Geometry check sheet. Reference: the model listing, model coordinates, mm. A direction names the side the tool comes from. Coordinates: 2 decimals unless noted, no trailing zeros. Order: outer loops, then holes, each group sorted by start corner. A loop starts at its lowest first (then second) coordinate and runs counter-clockwise, first axis right, second up. Notation, with made-up numbers: (-27.5, -8) - (17.5, -8) arc R6 cw to (17.5, 3) - close; hole circle Ø10 at (-32.75, 9.5). An arc over 180 degrees is marked (long way). Use CSV: the item, a comma, the result in double quotes. Start each with the question number.
1) Sectioned sample at C-C, the plane y = 7.5. Record the cut outline in (x, z), and give its area (3 significant figures).
2) Sectioned sample at A-A, the plane x = -277. Record the cut outline in (y, z), and give its area (3 significant figures).
3) Tool access check on faces 1 (the cylindrical face through (-283.885, -14.79, -25.186)), 2 (the flat face through (-289, -19, 0)), 3 (the cylindrical face through (-273.983, 20.23, -23.633)), 4 (the cylindrical face through (-273.983, 4.93, -23.633)), 5 (the flat face through (-285.529, 12.613, -50.347)). Record the directions out of +Z, -Z, +X, -X, +Y, -Y that give a thin tool (end or side, any length) a straight path to the whole face; none if there is none.
4) Depth check by flat-ended pin: P1, Ø20, axis at x = -282, y = -15.5, coming from the +Z side; P2, Ø6, axis at y = 6, z = -52.5, coming from the -X side; P3, Ø6, axis at y = -19, z = -35, coming from the -X side; P4, Ø19, axis at x = -272.5, z = -29, coming from the +Y side. Enter the tip coordinate at first touch or a pass-through.
5) Sectioned sample at D-D, the plane x = -293. Record the cut outline in (y, z), and give its area (3 significant figures).
6) Draft check along Y on faces 6 (the flat face through (-284, 0, -20)), 7 (the flat face through (-278, -40, -25)), 8 (the flat face through (-287, 25.3, -27)), 9 (the cylindrical face through (-264, -35, -23)). Enter one of: released by +Y, released by -Y, zero draft, split by the parting line, or undercut.
7) Sectioned sample at B-B, the plane z = -27. Record the cut outline in (x, y), and give its area (3 significant figures).
8) Thickness scan on probe 1 along Y at (x, z) = (-276.5, -12); probe 2 along Y at (x, z) = (-296.5, -4); probe 3 along Y at (x, z) = (-298.5, 1). Record the ranges inside material, lowest first. Write a range as [from, to].
Autodesk Inventor part; units mm, degrees
ref_plane "YZ Plane" through (0, 0, 0) normal (1, 0, 0) x (0, 1, 0)
ref_plane "XZ Plane" through (0, 0, 0) normal (0, 1, 0) x (-1, 0, 0)
ref_plane "XY Plane" through (0, 0, 0) normal (0, 0, 1) x (1, 0, 0)
sketch "Sketch1" plane through (0, 0, 0) normal (0, 1, 0) x (-1, 0, 0)
  circle A0 centre (0, 0) radius 285
  circle A1 centre (0, 0) radius 295
  circle A2 centre (0, 0) radius 275
  circle A3 centre (0, 0) radius 305
  line L0 (0, 0) -> (300.3664, -52.9627)
  line L1 (0, 0) -> (305, 0)
  point P0 (275, 0)
  point P1 (270.8221, -47.7532)
  dimension "d1" = 590
  dimension "d5" = 10
  dimension "d6" = 10
  dimension "d7" = 10
  dimension "d8" = 10
extrude "Extrusion1" add sketch "Sketch1" along normal blind 10 contours L1 A1 L0 A0 | A0 L0 A2 L1 | L1 A3 L0 A1 picked at (291.5003, -5.7176) picked at (281.3509, -10.8537) picked at (297.9408, -46.5324)
sketch "Sketch2" plane through (0, 10, 0) normal (0, 1, 0) x (1, 0, 0)
  arc A0 (-270.8221, 47.7532) -> (-275, 0) centre (0, 0) ccw
  line L0 (-270.8221, 47.7532) -> (-300.3664, 52.9627)
  arc A1 (-300.3664, 52.9627) -> (-305, 0) centre (0, 0) ccw
  line L1 (-305, 0) -> (-275, 0)
  circle A2 centre (0, 0) radius 295
  circle A3 centre (0, 0) radius 285
  circle A4 centre (0, 0) radius 294.7
  circle A5 centre (0, 0) radius 285.3
  point P0 (-285, 0)
  point P1 (-280.6702, 49.4897)
  point P2 (-290.5183, 51.2262)
  point P3 (-295, 0)
  point P4 (-285.3, 0)
  point P5 (-280.9657, 49.5418)
  point P6 (-290.2228, 51.1741)
  point P7 (-294.7, 0)
  dimension "d11" = 10
  dimension "d12" = 590
  dimension "d26" = 0.3
  dimension "d27" = 0.3
extrude "Extrusion2" add sketch "Sketch2" along normal blind 5.3 contours A5 L1 A4 L0 picked at (-291.2396, 11.2413)
sketch "Sketch3" plane through (0, 15.3, 0) normal (0, 1, 0) x (1, 0, 0)
  line L0 (-290.2228, 51.1741) -> (-300.3664, 52.9627)
  arc A0 (-300.3664, 52.9627) -> (-305, 0) centre (0, 0) ccw
  line L1 (-305, 0) -> (-294.7, 0)
  line L2 (-280.9657, 49.5418) -> (-290.2228, 51.1741)
  line L3 (-294.7, 0) -> (-285.3, 0)
  line L4 (-285.3, 0) -> (-275, 0)
  arc A1 (-270.8221, 47.7532) -> (-275, 0) centre (0, 0) ccw
  line L5 (-270.8221, 47.7532) -> (-280.9657, 49.5418)
  circle A2 centre (0, 0) radius 305
  circle A3 centre (0, 0) radius 275
  line L6 (0, 0) -> (-304.7097, -13.3039)
  line L7 (0, 0) -> (-297.7703, 66.0141)
  arc A4 (-300.3664, 52.9627) -> (-305, 0) centre (0, 0) ccw
  arc A5 (-270.8221, 47.7532) -> (-275, 0) centre (0, 0) ccw
  line L8 (-290.2228, 51.1741) -> (-300.3664, 52.9627)
  line L9 (-305, 0) -> (-294.7, 0)
  line L10 (-285.3, 0) -> (-275, 0)
  line L11 (-270.8221, 47.7532) -> (-280.9657, 49.5418)
  arc A6 (-290.2228, 51.1741) -> (-294.7, 0) centre (0, 0) ccw
  arc A7 (-280.9657, 49.5418) -> (-285.3, 0) centre (0, 0) ccw
  arc A8 (-290.2228, 51.1741) -> (-294.7, 0) centre (0, 0) ccw
  arc A9 (-280.9657, 49.5418) -> (-285.3, 0) centre (0, 0) ccw
  arc A10 (-290.2228, 51.1741) -> (-294.7, 0) centre (0, 0) ccw
  arc A11 (-280.9657, 49.5418) -> (-285.3, 0) centre (0, 0) ccw
  point P0 (-270.8221, 47.7532)
  point P1 (-268.4814, 59.5209)
  point P2 (-305, 0)
  point P3 (-274.7383, -11.9953)
  point P4 (-305, 0)
  point P5 (-300.3664, 52.9627)
  point P6 (-305, 0)
  point P7 (-270.8221, 47.7532)
  dimension "d23" = 2.5
  dimension "d28" = 2.5
extrude "Extrusion3" add sketch "Sketch3" along normal blind 10 contours A6 L1 A0 L0 | L0 A2 L7 A3 L5 L2 | L2 A7 L3 A6 | L5 A1 L4 A7 | L3 L4 A3 L6 A2 L1
sketch "Sketch4" plane through (0, 0, 0) normal (0, -1, 0) x (1, 0, 0)
  arc A0 (-275, 0) -> (-270.8221, -47.7532) centre (0, 0) ccw
  line L0 (-305, 0) -> (-275, 0)
  arc A1 (-305, 0) -> (-300.3664, -52.9627) centre (0, 0) ccw
  line L1 (-270.8221, -47.7532) -> (-300.3664, -52.9627)
  circle A2 centre (0, 0) radius 285
  circle A3 centre (0, 0) radius 295
  point P0 (-295, 0)
  point P1 (-290.5183, -51.2262)
  point P2 (-280.6702, -49.4897)
  point P3 (-285, 0)
  dimension "d17" = 10
  dimension "d18" = 590
extrude "Extrusion4" add sketch "Sketch4" along normal blind 30 contours A2 L1 A3 L0 picked at (-291.3396, -11.2413)
sketch "Sketch5" plane through (0, -30, 0) normal (0, -1, 0) x (1, 0, 0)
  arc A0 (-295, 0) -> (-290.5183, -51.2262) centre (0, 0) ccw
  line L0 (-290.5183, -51.2262) -> (-280.6702, -49.4897)
  arc A1 (-285, 0) -> (-280.6702, -49.4897) centre (0, 0) ccw
  line L1 (-285, 0) -> (-295, 0)
  arc A2 (-295, 0) -> (-290.5183, -51.2262) centre (0, 0) ccw
  line L2 (-305, 0) -> (-295, 0)
  arc A3 (-305, 0) -> (-300.3664, -52.9627) centre (0, 0) ccw
  line L3 (-290.5183, -51.2262) -> (-300.3664, -52.9627)
  line L4 (-270.8221, -47.7532) -> (-280.6702, -49.4897)
  arc A4 (-275, 0) -> (-270.8221, -47.7532) centre (0, 0) ccw
  line L5 (-285, 0) -> (-275, 0)
  arc A5 (-305, 0) -> (-300.3664, -52.9627) centre (0, 0) ccw
  arc A6 (-275, 0) -> (-270.8221, -47.7532) centre (0, 0) ccw
  arc A7 (-285, 0) -> (-280.6702, -49.4897) centre (0, 0) ccw
  arc A8 (-295, 0) -> (-290.5183, -51.2262) centre (0, 0) ccw
  line L6 (-305, 0) -> (-295, 0)
  line L7 (-290.5183, -51.2262) -> (-300.3664, -52.9627)
  arc A9 (-285, 0) -> (-280.6702, -49.4897) centre (0, 0) ccw
  line L8 (-270.8221, -47.7532) -> (-280.6702, -49.4897)
  line L9 (-285, 0) -> (-275, 0)
  arc A10 (-295, 0) -> (-290.5183, -51.2262) centre (0, 0) ccw
  circle A11 centre (0, 0) radius 265
  line L10 (0, 0) -> (-305, 0)
  line L11 (0, 0) -> (-300.3664, -52.9627)
  point P0 (-290.5183, -51.2262)
  point P1 (-260.9741, -46.0168)
  point P2 (-265, 0)
  dimension "d25" = 30
extrude "Extrusion5" add sketch "Sketch5" along normal blind 10 contours L1 A1 L0 A0 | L5 A4 L4 A1 | L10 A11 L11 A4
equation "\"d27\" = d26"
equation "\"d28\" = d23"
properties part number "Moving Caoursel base Clip" material "PLA Plastic"
Evaluation:
1,outline,"(-305, 0) arc R305 ccw to (-300.37, -52.96) - (-270.82, -47.75) arc R275 cw to (-275, 0) - close"
1,area,"1,520 mm²"
2,outline,"(-40, -48.84) - (-30, -48.84) - (-30, 0) - (-40, 0) - close; (0, -48.84) - (10, -48.84) - (10, 0) - (0, 0) - close; (15.3, -61.41) - (25.3, -61.41) - (25.3, 12.09) - (15.3, 12.09) - close"
2,area,"1,710 mm²"
3,face 1,"+Z, +X"
3,face 2,"+Z, +X, -X, -Y"
3,face 3,"+X, +Y"
3,face 4,"+Z, +X, +Y"
3,face 5,"-Z, +X, -Y"
4,P1,"z = 0"
4,P2,"x = -300.96"
4,P3,"x = -293.26"
4,P4,"y = 25.3"
5,outline,"(-40, -34.29) - (0, -34.29) - (0, -51.66) - (10, -51.66) - (10, -31.61) - (15.3, -31.61) - (15.3, -64.96) - (25.3, -64.96) - (25.3, 12.79) - (15.3, 12.79) - (15.3, 0) - (-40, 0) - close"
5,area,"2,830 mm²"
6,face 6,"undercut"
6,face 7,"released by -Y"
6,face 8,"released by +Y"
6,face 9,"zero draft"
7,outline,"(-303.8, 0) - (-293.76, 0) - (-293.76, -40) - (-263.62, -40) - (-263.62, -30) - (-283.72, -30) - (-283.72, 0) - (-273.67, 0) - (-273.67, 10) - (-284.02, 10) - (-284.02, 15.3) - (-273.67, 15.3) - (-273.67, 25.3) - (-303.8, 25.3) - (-303.8, 15.3) - (-293.46, 15.3) - (-293.46, 10) - (-303.8, 10) - close"
7,area,"1,260 mm²"
8,probe 1,"[-40, -30], [0, 10], [15.3, 25.3]"
8,probe 2,"[0, 10], [15.3, 25.3]"
8,probe 3,"[15.3, 25.3]"
